from build123d import *

# Parameters (mm, degrees)
F0_W     = 60
F0_H     = 60
F1_DEPTH = 3.175
F2_W     = 10
F2_H     = 3.175
F3_DEPTH = 3.176
F4_R     = 5


# Not quite as in the source:
# - a length typed as a fraction of an inch, garbled in the dataset ("3 / 203.2 mm" for 3/8 in), is restored


with BuildPart() as f1:
    # F0 (on Front) → F1 (new body)
    with BuildSketch(Plane.XZ):
        Rectangle(F0_W, F0_H)
    extrude(amount=F1_DEPTH)

    # F2 (on face) → F3 (cut, through all)
    with BuildSketch(Plane.XZ.offset(3.175)):
        with Locations((-20, -15.875)):
            Rectangle(F2_W, F2_H)
        with Locations((0, -15.875)):
            Rectangle(F2_W, F2_H)
        with Locations((20, -15.875)):
            Rectangle(F2_W, F2_H)
        with Locations((-20, -9.525)):
            Rectangle(F2_W, F2_H)
        with Locations((0, -9.525)):
            Rectangle(F2_W, F2_H)
        with Locations((20, -9.525)):
            Rectangle(F2_W, F2_H)
        with Locations((-20, -3.175)):
            Rectangle(F2_W, F2_H)
        with Locations((0, -3.175)):
            Rectangle(F2_W, F2_H)
        with Locations((20, -3.175)):
            Rectangle(F2_W, F2_H)
        with Locations((-20, 3.175)):
            Rectangle(F2_W, F2_H)
        with Locations((0, 3.175)):
            Rectangle(F2_W, F2_H)
        with Locations((20, 3.175)):
            Rectangle(F2_W, F2_H)
        with Locations((-20, 9.525)):
            Rectangle(F2_W, F2_H)
        with Locations((0, 9.525)):
            Rectangle(F2_W, F2_H)
        with Locations((20, 9.525)):
            Rectangle(F2_W, F2_H)
        with Locations((-20, 15.875)):
            Rectangle(F2_W, F2_H)
        with Locations((0, 15.875)):
            Rectangle(F2_W, F2_H)
        with Locations((20, 15.875)):
            Rectangle(F2_W, F2_H)
    extrude(amount=-F3_DEPTH, mode=Mode.SUBTRACT)

    # F4
    f4_edges = [f1.edges().sort_by_distance(p)[0] for p in [
        (-30, -1.5875, 30),
        (30, -1.5875, 30),
        (-30, -1.5875, -30),
        (30, -1.5875, -30),
    ]]
    fillet(f4_edges, radius=F4_R)


solid = f1.part
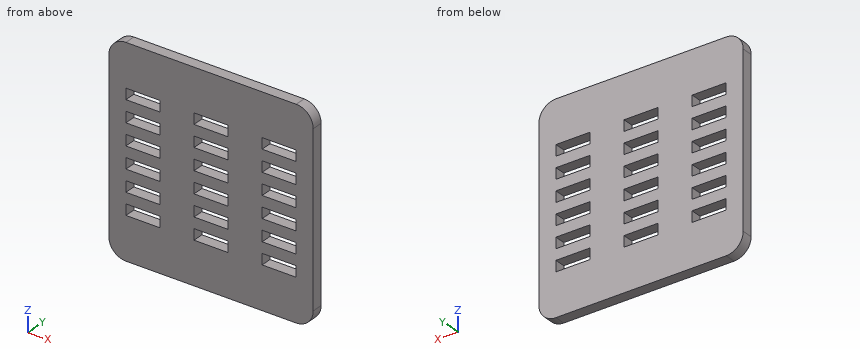
Model file for the job. Use its own axes, mm. Give positions to 0.01 mm unless a question says otherwise; leave off trailing zeros. Order: outer loops, then holes, each group sorted by start corner. A loop starts at its lowest first (then second) coordinate and runs counter-clockwise, first axis right, second up. Notation, with made-up numbers: M 79,-26 L 124,-26 A24 cw 124,-8 Z; hole C -26,26 d8. An arc over 180 degrees is marked long. Put each result on its own line as item: value. Start each with the question number.
(1) Band-saw the part on C-C on y = -2.35. Count the separate pieces of the cut face and the enclosed holes in it, then the cut area to 3 significant figures.
(2) Band-saw the part on B-B on x = -4. Give the cut face in (y, z) (1 decimal), then the cut area to 3 significant figures.
(3) Drill centre lines: L1, parallel to X at y = -0.8, z = -10.5; L2, parallel to Z at x = 27.5, y = -0.7; L3, parallel to Z at x = 27, y = -0.7. Where is each one in solid material? Low to high. Write a range as [from, to].
(4) Band-saw the part on A-A on z = -15.5. Give the cut face in (x, y) (3 decimals).
Results below:
1. separate pieces: 1
1. enclosed holes: 18
1. area: 3,010 mm2
2. outline: M -3.2,-30 L 0,-30 L 0,-17.5 L -3.2,-17.5 Z; M -3.2,-14.3 L 0,-14.3 L 0,-11.1 L -3.2,-11.1 Z; M -3.2,-7.9 L 0,-7.9 L 0,-4.8 L -3.2,-4.8 Z; M -3.2,-1.6 L 0,-1.6 L 0,1.6 L -3.2,1.6 Z; M -3.2,4.8 L 0,4.8 L 0,7.9 L -3.2,7.9 Z; M -3.2,11.1 L 0,11.1 L 0,14.3 L -3.2,14.3 Z; M -3.2,17.5 L 0,17.5 L 0,30 L -3.2,30 Z
2. area: 130 mm2
3. L1: x = [-30, -25], [-15, -5], [5, 15], [25, 30]
3. L2: z = [-29.33, 29.33]
3. L3: z = [-29.58, 29.58]
4. outline: M -30,-3.175 L -25,-3.175 L -25,0 L -30,0 Z; M -15,-3.175 L -5,-3.175 L -5,0 L -15,0 Z; M 5,-3.175 L 15,-3.175 L 15,0 L 5,0 Z; M 25,-3.175 L 30,-3.175 L 30,0 L 25,0 Z
